from build123d import *

# Parameters (mm, degrees)
F1_DEPTH = 12.5
F2_R     = 0.2


with BuildPart() as f1:
    # F0 (on Top) → F1 (new body)
    with BuildSketch(Plane.XY):
        Polygon((0, 50), (0, 0), (74.3, 0), (24.3, 50), align=None)
    extrude(amount=-F1_DEPTH)

    # F2
    f2_edges = [f1.edges().sort_by_distance(p)[0] for p in [
        (12.15, 50, 0),
        (0, 25, 0),
        (37.15, 0, 0),
        (49.3, 25, 0),
        (12.15, 50, -12.5),
        (0, 25, -12.5),
        (37.15, 0, -12.5),
        (49.3, 25, -12.5),
    ]]
    fillet(f2_edges, radius=F2_R)


solid = f1.part
The model under review builds one solid part; all positions refer to its coordinate system, in mm. Round coordinates to 2 decimals unless told otherwise and drop trailing zeros. Loops run counter-clockwise (first coordinate to the right, second up) from the corner with the lowest first, then second, coordinate; pieces in that order, holes last. Notation, with made-up numbers: (64, -28) -> (120, -28) arc R18 cw to (120, -7) -> close; hole circle Ø4 at (89, 48.5). An arc over 180 degrees is marked (long way). Return JSON: item names as keys, results as strings.
(1) For pin 1 (1 mm diameter, centred on y = 41, z = -6, fed in from +X); pin 2 (5 mm diameter, centred on y = 20, z = -8, fed in from +X), all flat-tipped, find the tip position at first contact; note any pin that passes through.
Solved:
{"pin 1": "x = 33.8", "pin 2": "x = 56.8"}
(2) The part is to be moulded in two halves that separate along Y. For faces 1 (the flat face through (37, 0, -6)), 2 (the flat face through (0, 25, -6)), 3 (the flat face through (12, 50, -6)), say which applies: released by +Y, released by -Y, zero draft, split by the parting line, or undercut.
Solved:
{"face 1": "released by -Y", "face 2": "zero draft", "face 3": "released by +Y"}
(3) Add section A-A on z = -10.5. Write out the cut boundary in (x, y), plus the area to 4 significant figures.
Solved:
{"outline": "(0, 0) -> (74.3, 0) -> (24.3, 50) -> (0, 50) -> close", "area": "2,465 mm2"}
(4) For line 1 (Y direction, x = 67.5, z = -2.5); line 2 (Y direction, x = 54, z = -7.75); line 3 (X direction, y = 32, z = -5.25), list the stretches that pass through material, from the lowest coordinate up.
Solved:
{"line 1": "0 to 6.8", "line 2": "0 to 20.3", "line 3": "0 to 42.3"}
